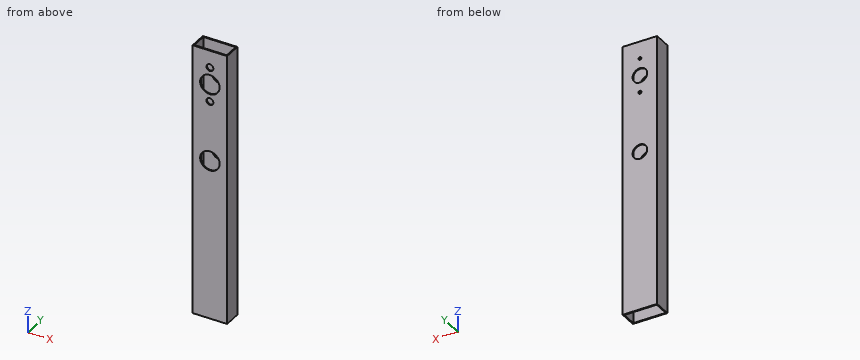
```python
from build123d import *

# Parameters (mm, degrees)
SKETCH1_W           = 50.8
SKETCH1_H           = 25.4
SKETCH1_W_2         = 47.625
SKETCH1_H_2         = 22.225
BOSS_EXTRUDE1_DEPTH = 401.32
SKETCH2_R           = 10.795
CUT_EXTRUDE1_DEPTH  = 2.54
SKETCH3_R           = 10.795
CUT_EXTRUDE2_DEPTH  = 4.92
SKETCH5_R           = 14.351
CUT_EXTRUDE3_DEPTH  = 12.7
SKETCH6_R           = 14.351
CUT_EXTRUDE4_DEPTH  = 12.7
SKETCH7_R           = 2.159
CUT_EXTRUDE5_DEPTH  = 2.54
SKETCH9_R           = 5.08
CUT_EXTRUDE6_DEPTH  = 2.54
SKETCH10_R          = 2.286
CUT_EXTRUDE7_DEPTH  = 2.54
SKETCH11_R          = 5.08
CUT_EXTRUDE8_DEPTH  = 2.54


with BuildPart() as part:
    # Sketch1 → Boss-Extrude1 (new body)
    with BuildSketch(Plane.XY):
        with Locations((25.4, 12.7)):
            Rectangle(SKETCH1_W, SKETCH1_H)
        with Locations((25.4, 12.7)):
            Rectangle(SKETCH1_W_2, SKETCH1_H_2, mode=Mode.SUBTRACT)
    extrude(amount=BOSS_EXTRUDE1_DEPTH)

    # Sketch2 → Cut-Extrude1 (cut)
    with BuildSketch(Plane(origin=(0, 25.4, 0), x_dir=(1, 0, 0), z_dir=(0, 1, 0))):
        with Locations(Location((25.4, -236.22, 0), (0, 0, 270))):
            Circle(SKETCH2_R)
    extrude(amount=-CUT_EXTRUDE1_DEPTH, mode=Mode.SUBTRACT)

    # Sketch3 → Cut-Extrude2 (cut)
    with BuildSketch(Plane(origin=(0, 25.4, 0), x_dir=(1, 0, 0), z_dir=(0, 1, 0))):
        with Locations(Location((25.4, -350.52, 0), (0, 0, 270))):
            Circle(SKETCH3_R)
    extrude(amount=-CUT_EXTRUDE2_DEPTH, mode=Mode.SUBTRACT)

    # Sketch5 → Cut-Extrude3 (cut)
    with BuildSketch(Plane(origin=(0, 1.5875, 0), x_dir=(1, 0, 0), z_dir=(0, 1, 0))):
        with Locations(Location((25.4, -236.22, 0), (0, 0, 270))):
            Circle(SKETCH5_R)
    extrude(amount=-CUT_EXTRUDE3_DEPTH, mode=Mode.SUBTRACT)

    # Sketch6 → Cut-Extrude4 (cut)
    with BuildSketch(Plane(origin=(0, 1.5875, 0), x_dir=(1, 0, 0), z_dir=(0, 1, 0))):
        with Locations(Location((25.4, -350.52, 0), (0, 0, 270))):
            Circle(SKETCH6_R)
    extrude(amount=-CUT_EXTRUDE4_DEPTH, mode=Mode.SUBTRACT)

    # Sketch7 → Cut-Extrude5 (cut)
    with BuildSketch(Plane(origin=(0, 25.4, 0), x_dir=(1, 0, 0), z_dir=(0, 1, 0))):
        with Locations(Location((25.4, -375.92, 0), (0, 0, 270))):
            Circle(SKETCH7_R)
    extrude(amount=-CUT_EXTRUDE5_DEPTH, mode=Mode.SUBTRACT)

    # Sketch9 → Cut-Extrude6 (cut)
    with BuildSketch(Plane(origin=(0, 1.5875, 0), x_dir=(1, 0, 0), z_dir=(0, 1, 0))):
        with Locations(Location((25.4, -375.92, 0), (0, 0, 270))):
            Circle(SKETCH9_R)
    extrude(amount=-CUT_EXTRUDE6_DEPTH, mode=Mode.SUBTRACT)

    # Sketch10 → Cut-Extrude7 (cut)
    with BuildSketch(Plane(origin=(0, 25.4, 0), x_dir=(1, 0, 0), z_dir=(0, 1, 0))):
        with Locations(Location((25.4, -325.12, 0), (0, 0, 270))):
            Circle(SKETCH10_R)
    extrude(amount=-CUT_EXTRUDE7_DEPTH, mode=Mode.SUBTRACT)

    # Sketch11 → Cut-Extrude8 (cut)
    with BuildSketch(Plane(origin=(0, 1.5875, 0), x_dir=(1, 0, 0), z_dir=(0, 1, 0))):
        with Locations(Location((25.4, -325.12, 0), (0, 0, 270))):
            Circle(SKETCH11_R)
    extrude(amount=-CUT_EXTRUDE8_DEPTH, mode=Mode.SUBTRACT)


solid = part.part
```
Part model, mm, in its own coordinate system. Round coordinates to 2 decimals unless told otherwise and drop trailing zeros. Order: outer loops, then holes, each group sorted by start corner. A loop starts at its lowest first (then second) coordinate and runs counter-clockwise, first axis right, second up. Notation, with made-up numbers: M -1.5,5 L 15.5,5 A20 cw 15.5,10 Z; hole C -31,47.25 d5. An arc over 180 degrees is marked long. Answer in a Markdown table with one row per item. Add a question column.
Q1. Cut at B-B on x = 45. Give the cut face in (y, z), and give its area (3 significant figures).
Q2. Cut at D-D on z = 62. Give the cut face in (x, y).
Q3. Cut at C-C on y = 13. Give the cut face in (x, z), and give its area (3 significant figures).
Q4. Pin check, flat tips, straight feed: pin 1 (13 mm diameter, centred on x = 25.4, z = 236.22, fed in from +Y); pin 2 (5 mm diameter, centred on x = 25.4, z = 375.92, fed in from -Y). Stop position of each tip, or through.
Q5. Cut at A-A on z = 350.52. Give the cut face in (x, y) (1 decimal), and give its area (3 significant figures).
Q6. Wall check: L1, parallel to Z at x = 25, y = 24.5; L2, parallel to Y at x = 27.5, z = 208.5; L3, parallel to X at y = 0.9, z = 325.12. Give the ranges that are in metal, low to high. Write a range as from..to.
Established:
| question | item | result |
|---|---|---|
| 1 | outline | M 0,0 L 1.59,0 L 1.59,401.32 L 0,401.32 Z; M 23.81,0 L 25.4,0 L 25.4,401.32 L 23.81,401.32 Z |
| 1 | area | 1,270 mm2 |
| 2 | outline | M 0,0 L 50.8,0 L 50.8,25.4 L 0,25.4 Z; hole M 1.59,1.59 L 49.21,1.59 L 49.21,23.81 L 1.59,23.81 Z |
| 3 | outline | M 0,0 L 1.59,0 L 1.59,401.32 L 0,401.32 Z; M 49.21,0 L 50.8,0 L 50.8,401.32 L 49.21,401.32 Z |
| 3 | area | 1,270 mm2 |
| 4 | pin 1 | passes through |
| 4 | pin 2 | stops at y = 23.81 |
| 5 | outline | M 0,0 L 11,0 L 11,1.6 L 1.6,1.6 L 1.6,23.8 L 14.6,23.8 L 14.6,25.4 L 0,25.4 Z; M 36.2,23.8 L 49.2,23.8 L 49.2,1.6 L 39.8,1.6 L 39.8,0 L 50.8,0 L 50.8,25.4 L 36.2,25.4 Z |
| 5 | area | 152 mm2 |
| 6 | L1 | z = 0..225.43, 247.01..322.87, 327.37..339.73, 361.31..373.8, 378.04..401.32 |
| 6 | L2 | y = 0..1.59, 23.81..25.4 |
| 6 | L3 | x = 0..20.32, 30.48..50.8 |
